Can you work these out from the model? Positions are in its coordinate system, mm. A direction names the side the tool comes from. Give positions to 0.01 mm unless a question says otherwise; leave off trailing zeros. Order: outer loops, then holes, each group sorted by start corner. A loop starts at its lowest first (then second) coordinate and runs counter-clockwise, first axis right, second up. Notation, with made-up numbers: (80.25, -12) - (99.25, -12) arc R26 ccw to (99.25, 7) - close; hole circle Ø6 at (-31.5, 24). An arc over 180 degrees is marked (long way). Use one line per item in the form item = value. Start each with the question number.
1) Which directions (+Z, -Z, +X, -X, +Y, -Y) give clear straight access to the entire face, cutting with the end or side of a thin tool? Please do faces 5 (the cylindrical face through (-11.4, 34.5, 1.5)), 6 (the cylindrical face through (-15.926, -33.648, 4.972)).
2) For pin 1 (1.7 mm diameter, centred on x = -6.07, y = 46.37, fed in from +Z); pin 2 (4 mm diameter, centred on x = -13, y = -6.5, fed in from +Z); pin 3 (1.5 mm diameter, centred on x = -15, z = 5.5, fed in from -Y), each with a flat end and sliding along its axis, tell me the tip position at first contact or that it passes through.
3) Suppose I cut it at B-B, the plane y = 12.5. Write out the boundary of the cut face in (x, z), and give its area (3 significant figures).
4) Please list where these lines run through material, in increasing order: probe 1 along Z at (x, y) = (-39, -5.5); probe 2 along X at (y, z) = (-11, 0.5); probe 3 along X at (y, z) = (-12, 2.25).
5) Suppose I cut it at C-C, the plane x = -26. Write out the boundary of the cut face in (y, z), and give its area (3 significant figures).
6) We'd pull the mould along X, two halves only. Please class faces 1 (the cylindrical face through (-41.02, 28.44, 4.97)), 2 (the cylindrical face through (-56.406, 46.924, 1.521)), 3 (the cylindrical face through (-56.45, -12.07, 1.52)), 4 (the flat face through (-31, 15, 3)): released by +X, released by -X, zero draft, split by the parting line, or undercut.
7) Suppose I cut it at A-A, the plane z = 4.25. Write out the boundary of the cut face in (x, y).
```python
from build123d import *

# Parameters (mm, degrees)
BOSS_EXTRUDE1_DEPTH = 3
SKETCH3_R           = 1.6
SKETCH3_R_2         = 1.45
CUT_EXTRUDE1_DEPTH  = 89.191303006
SKETCH4_R           = 3.5
SKETCH4_R_2         = 1.45
BOSS_EXTRUDE2_DEPTH = 4


with BuildPart() as part:
    # Sketch2 → Boss-Extrude1 (new body)
    with BuildSketch(Plane.XY):
        with BuildLine():
            Line((-55.566838563, -38.131712133), (-5.566838563, -38.131712133))
            ThreePointArc((-5.566838563, -38.131712133), (-3.44551822, -37.253032477), (-2.566838563, -35.131712133))
            Line((-2.566838563, -35.131712133), (-2.566838563, 65.868287867))
            Line((-2.566838563, 65.868287867), (-58.566838563, 65.868287867))
            Line((-58.566838563, 65.868287867), (-58.566838563, -35.131712133))
            ThreePointArc((-58.566838563, -35.131712133), (-57.688158907, -37.253032477), (-55.566838563, -38.131712133))
        make_face()
    extrude(amount=BOSS_EXTRUDE1_DEPTH)

    # Sketch3 → Cut-Extrude1 (cut, through all)
    with BuildSketch(Plane.XY.offset(3)):
        with Locations((-50.566838563, 35.868287867)):
            Circle(SKETCH3_R)
        with Locations((-50.566838563, 5.868287867)):
            Circle(SKETCH3_R)
        with Locations(Location((-10.566838563, 5.868287867, 0), (0, 0, 180))):
            Circle(SKETCH3_R)
        with Locations(Location((-10.566838563, 35.868287867, 0), (0, 0, 180))):
            Circle(SKETCH3_R)
        with Locations((-40.566838563, 24.968287867)):
            Circle(SKETCH3_R_2)
        with Locations((-15.166838563, -30.231712133)):
            Circle(SKETCH3_R_2)
        with Locations((-6.066838563, 46.368287867)):
            Circle(SKETCH3_R_2)
        with Locations((-6.066838563, -11.631712133)):
            Circle(SKETCH3_R_2)
        with Locations(Location((-55.066838563, -11.631712133, 0), (0, 0, 180))):
            Circle(SKETCH3_R_2)
        with Locations(Location((-55.066838563, 46.368287867, 0), (0, 0, 180))):
            Circle(SKETCH3_R_2)
    extrude(amount=-CUT_EXTRUDE1_DEPTH, mode=Mode.SUBTRACT)

    # Sketch4 → Boss-Extrude2 (add)
    with BuildSketch(Plane.XY.offset(3)):
        with Locations((-40.566838563, 24.968287867)):
            Circle(SKETCH4_R)
        with Locations((-40.566838563, 24.968287867)):
            Circle(SKETCH4_R_2, mode=Mode.SUBTRACT)
        with Locations((-15.166838563, -30.231712133)):
            Circle(SKETCH4_R)
        with Locations((-15.166838563, -30.231712133)):
            Circle(SKETCH4_R_2, mode=Mode.SUBTRACT)
    extrude(amount=BOSS_EXTRUDE2_DEPTH)


solid = part.part
```
Result sheet:
q1.face_5 = +Z, -Z
q1.face_6 = +Z
q2.pin_1 = through
q2.pin_2 = 3
q2.pin_3 = -33.73
q3.outline = (-58.57, 0) - (-2.57, 0) - (-2.57, 3) - (-58.57, 3) - close
q3.area = 168 mm²
q4.probe_1 = 0 to 3
q4.probe_2 = -58.57 to -56.37, -53.76 to -7.37, -4.76 to -2.57
q4.probe_3 = -58.57 to -56.47, -53.66 to -7.47, -4.66 to -2.57
q5.outline = (-38.13, 0) - (65.87, 0) - (65.87, 3) - (-38.13, 3) - close
q5.area = 312 mm²
q6.face_1 = split by the parting line
q6.face_2 = undercut
q6.face_3 = undercut
q6.face_4 = zero draft
q7.outline = circle Ø7 at (-40.57, 24.97); circle Ø7 at (-15.17, -30.23); hole circle Ø2.9 at (-40.57, 24.97); hole circle Ø2.9 at (-15.17, -30.23)
